Source: CAD feature listing. Evaluate the final solid. Frame: model axes, mm. Face numbers are marked on the shaded views. A direction names the side the tool comes from. Coordinates: 2 decimals unless noted, no trailing zeros. Loops run counter-clockwise (first coordinate to the right, second up) from the corner with the lowest first, then second, coordinate; pieces in that order, holes last. Notation, with made-up numbers: (19, 39.25) -> (55, 39.25) arc R28 ccw to (55, 74.25) -> close; hole circle Ø4 at (-27.5, 20). An arc over 180 degrees is marked (long way). Answer as CSV lines item,"result".
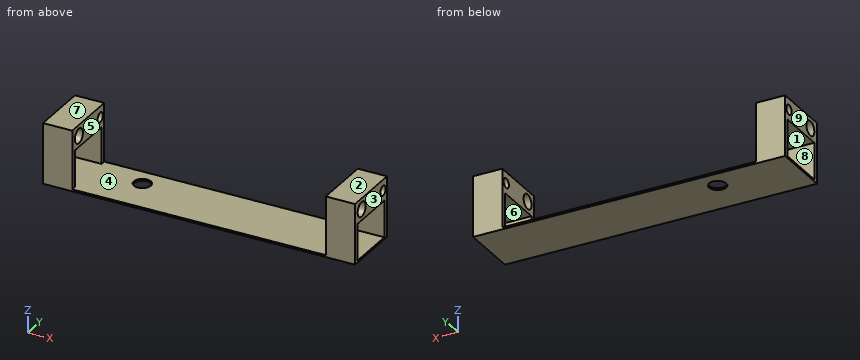
from build123d import *

# Parameters (mm, degrees)
SKETCH1_W           = 609.6
SKETCH1_H           = 76.2
SKETCH1_R           = 11.1125
BOSS_EXTRUDE1_DEPTH = 2.54
SKETCH2_W           = 38.1
SKETCH2_H           = 6.35
BOSS_EXTRUDE2_DEPTH = 76.2
SKETCH3_W           = 38.1
SKETCH3_H           = 76.2
BOSS_EXTRUDE3_DEPTH = 28.575
SKETCH4_R           = 6.35
SKETCH4_R_2         = 9.525
CUT_EXTRUDE1_DEPTH  = 610.6
SKETCH5_W           = 203.2
SKETCH5_H           = 76.2
CUT_EXTRUDE2_DEPTH  = 3.54


with BuildPart() as part:
    # Sketch1 → Boss-Extrude1 (new body)
    with BuildSketch(Plane.XY):
        with Locations((0, 21.113121982)):
            Rectangle(SKETCH1_W, SKETCH1_H)
        with Locations((0, 33.813121982)):
            Circle(SKETCH1_R, mode=Mode.SUBTRACT)
    extrude(amount=BOSS_EXTRUDE1_DEPTH)

    # Sketch2 → Boss-Extrude2 (add)
    with BuildSketch(Plane.XY.offset(2.54)):
        with Locations((-82.55, 56.038121982)):
            Rectangle(SKETCH2_W, SKETCH2_H)
        with Locations((-82.55, -13.811878018)):
            Rectangle(SKETCH2_W, SKETCH2_H)
        with Locations((285.75, 56.038121982)):
            Rectangle(SKETCH2_W, SKETCH2_H)
        with Locations((285.75, -13.811878018)):
            Rectangle(SKETCH2_W, SKETCH2_H)
    extrude(amount=BOSS_EXTRUDE2_DEPTH)

    # Sketch3 → Boss-Extrude3 (add)
    with BuildSketch(Plane.XY.offset(78.74)):
        with Locations((-82.55, 21.113121982)):
            Rectangle(SKETCH3_W, SKETCH3_H)
        with Locations((285.75, 21.113121982)):
            Rectangle(SKETCH3_W, SKETCH3_H)
    extrude(amount=-BOSS_EXTRUDE3_DEPTH)

    # Sketch4 → Cut-Extrude1 (cut, through all)
    with BuildSketch(Plane(origin=(304.8, 0, 0), x_dir=(0, 0, -1), z_dir=(1, 0, 0))):
        with Locations((-64.4525, 49.688121982)):
            Circle(SKETCH4_R)
        with Locations((-64.4525, -1.111878018)):
            Circle(SKETCH4_R_2)
    extrude(amount=-CUT_EXTRUDE1_DEPTH, mode=Mode.SUBTRACT)

    # Sketch5 → Cut-Extrude2 (cut, through all)
    with BuildSketch(Plane.XY.offset(2.54)):
        with Locations((-203.2, 21.113121982)):
            Rectangle(SKETCH5_W, SKETCH5_H)
    extrude(amount=-CUT_EXTRUDE2_DEPTH, mode=Mode.SUBTRACT)


solid = part.part
(1) Pin query (flat end, axial travel): pin 1 Ø1 at (x, y) = (199.5, -7.5) entering from +Z. Return the tip coordinate at first contact, or that it passes through.
Computed values:
pin 1,"z = 2.54"
(2) Draft query along Z for the marked faces 6, 7, 8 and 9. Return one class per face: released by +Z, released by -Z, zero draft, split by the parting line, or undercut.
Computed values:
face 6,"undercut"
face 7,"released by +Z"
face 8,"undercut"
face 9,"zero draft"
(3) Cut plane C-C (x = 51.5). Return the cut outline in (y, z).
Computed values:
outline,"(-16.99, 0) -> (59.21, 0) -> (59.21, 2.54) -> (-16.99, 2.54) -> close"
(4) Cut plane B-B (z = 25). Return the cut outline in (x, y).
Computed values:
outline,"(-101.6, -16.99) -> (-63.5, -16.99) -> (-63.5, -10.64) -> (-101.6, -10.64) -> close; (-101.6, 52.86) -> (-63.5, 52.86) -> (-63.5, 59.21) -> (-101.6, 59.21) -> close; (266.7, -16.99) -> (304.8, -16.99) -> (304.8, -10.64) -> (266.7, -10.64) -> close; (266.7, 52.86) -> (304.8, 52.86) -> (304.8, 59.21) -> (266.7, 59.21) -> close"
(5) Access query for the marked faces 1, 2, 3, 4 and 5. Directions: +Z, -Z, +X, -X, +Y, -Y. A direction counts if a zero-diameter tool reaches every point of the face in a straight line with its end or side. Return the directions, or none.
Computed values:
face 1,"+X, -X"
face 2,"+Z, +X, -X, +Y, -Y"
face 3,"+Z, -Z, +X, +Y, -Y"
face 4,"none"
face 5,"+Z, +Y, -Y"
(6) Material intervals for L1, parallel to X at y = 49, z = 72; L2, parallel to Z at x = 271.5, y = 14 (3 decimals); L3, parallel to Y at x = 0, z = 1, sorted ascending. Write a range as [from, to].
Computed values:
L1,"[-101.6, -63.5], [266.7, 304.8]"
L2,"[0, 2.54], [50.165, 78.74]"
L3,"[-16.99, 22.7], [44.93, 59.21]"
(7) Cut plane A-A (x = 0). Return the cut outline in (y, z).
Computed values:
outline,"(-16.99, 0) -> (22.7, 0) -> (22.7, 2.54) -> (-16.99, 2.54) -> close; (44.93, 0) -> (59.21, 0) -> (59.21, 2.54) -> (44.93, 2.54) -> close"
